```python
from build123d import *

# Parameters (mm, degrees)
F0_W     = 253
F0_H     = 17.5
F1_DEPTH = 5
F2_D     = 4
F0_H_2   = 5
F3_DEPTH = 40
F4_DEPTH = 5
F5_D     = 4


with BuildPart() as f1:
    # F0 (on Top) → F1 (new body)
    with BuildSketch(Plane.XY):
        with Locations((0.5246251822, -26.25)):
            Rectangle(F0_W, F0_H)
    extrude(amount=F1_DEPTH)

    # F2 (through all)
    with Locations(Plane(origin=(0, 0, 0), x_dir=(1, 0, 0), z_dir=(0, 0, -1))):
        with Locations((-114.9753748178, 0), (-114.9753748178, 30), (119.0246251822, 30), (119.0246251822, 0)):
            Hole(F2_D / 2)

    # F0 (on Top) → F3 (join)
    with BuildSketch(Plane.XY):
        with Locations((0.5246251822, -15)):
            Rectangle(F0_W, F0_H_2)
    extrude(amount=F3_DEPTH)

    # F0 (on Top) → F4 (join)
    with BuildSketch(Plane.XY):
        with Locations((0.5246251822, -3.75)):
            Rectangle(F0_W, F0_H)
    extrude(amount=F4_DEPTH)

    # F5 (through all)
    with Locations(Plane(origin=(0, 0, 0), x_dir=(1, 0, 0), z_dir=(0, 0, -1))):
        with Locations((-114.9753748178, 0), (119.0246251822, 0)):
            Hole(F5_D / 2)


solid = f1.part
```
CAD build for the part. Positions are in the model's coordinates, mm. A direction names the side the tool comes from. Round coordinates to 2 decimals unless told otherwise and drop trailing zeros. Write each loop counter-clockwise with the first axis right and the second up, starting at its lowest first coordinate (ties: lowest second). Pieces come first, ordered by that corner, then holes. Notation, with made-up numbers: (-36, 56) - (15, 56) arc R10 ccw to (15, 67) - close; hole circle Ø7 at (57, 85). An arc over 180 degrees is marked (long way). Return JSON: item names as keys, results as strings. Group by question number.
Item 1: Flat gauge pins, fed straight in: pin 1 Ø1 at (x, z) = (101, 24) entering from +Y; pin 2 Ø2.5 at (x, y) = (-114.98, 0) entering from -Z; pin 3 Ø5 at (x, y) = (119.02, -30) entering from +Z; pin 4 Ø1.5 at (x, z) = (52, 21.5) entering from -Y. Where does each tip first touch, or does it go through?
Item 2: Probe probe 1 along X at (y, z) = (-30, 1.7); probe 2 along Y at (x, z) = (-66.5, 21); probe 3 along Z at (x, y) = (-87, -23). List the from-to ranges inside material, lowest first.
Item 3: Band-saw the part on A-A on x = -22. List the corners of the cut face in (y, z), plus the area to 3 significant figures.
Item 4: Band-saw the part on B-B on z = 37.5. List the corners of the cut face in (x, y), plus the area to 4 significant figures.
Item 5: Mould opens along X. For faces 1 (the face through (117.117, -0.601, 2.535)), 2 (the face through (-125.975, -15, 12)), 3 (the face through (-1, 5, 2)), 4 (the face through (-116.883, -0.601, 2.535)) say: +X half, -X half, draft (parallel to the pull), parting line (faces both ways), or undercut.
Item 6: 3-axis set-ups, long thin cutter, end or side, ignore diameter. For faces 5 (the face through (-1, -4, 5)), 6 (the face through (-1, -15, 40)), 7 (the face through (-1, -17.5, 22)): which of +Z, -Z, +X, -X, +Y, -Y reach the whole face in a straight line?
Item 7: Band-saw the part on C-C on y = -25. List the corners of the cut face in (x, z).
Resolved:
{
 "1": {"pin 1": "stops at y = -12.5", "pin 2": "passes through", "pin 3": "stops at z = 5", "pin 4": "stops at y = -17.5"},
 "2": {"probe 1": "x = -125.98 to -116.98, -112.98 to 117.02, 121.02 to 127.02", "probe 2": "y = -17.5 to -12.5", "probe 3": "z = 0 to 5"},
 "3": {"outline": "(-35, 0) - (5, 0) - (5, 5) - (-12.5, 5) - (-12.5, 40) - (-17.5, 40) - (-17.5, 5) - (-35, 5) - close", "area": "375 mm²"},
 "4": {"outline": "(-125.98, -17.5) - (127.02, -17.5) - (127.02, -12.5) - (-125.98, -12.5) - close", "area": "1,265 mm²"},
 "5": {"face 1": "undercut", "face 2": "-X half", "face 3": "draft", "face 4": "undercut"},
 "6": {"face 5": "+Z, +X, -X, +Y", "face 6": "+Z, +X, -X, +Y, -Y", "face 7": "+Z, +X, -X, -Y"},
 "7": {"outline": "(-125.98, 0) - (127.02, 0) - (127.02, 5) - (-125.98, 5) - close"}
}
